Design review of the part shown in the three views and the two pictorial views. Dimensions are in mm from the part's minimum x, y and z. Give positions to 0.01 mm unless a question says otherwise; leave off trailing zeros. Loops run counter-clockwise (first coordinate to the right, second up) from the corner with the lowest first, then second, coordinate; pieces in that order, holes last.
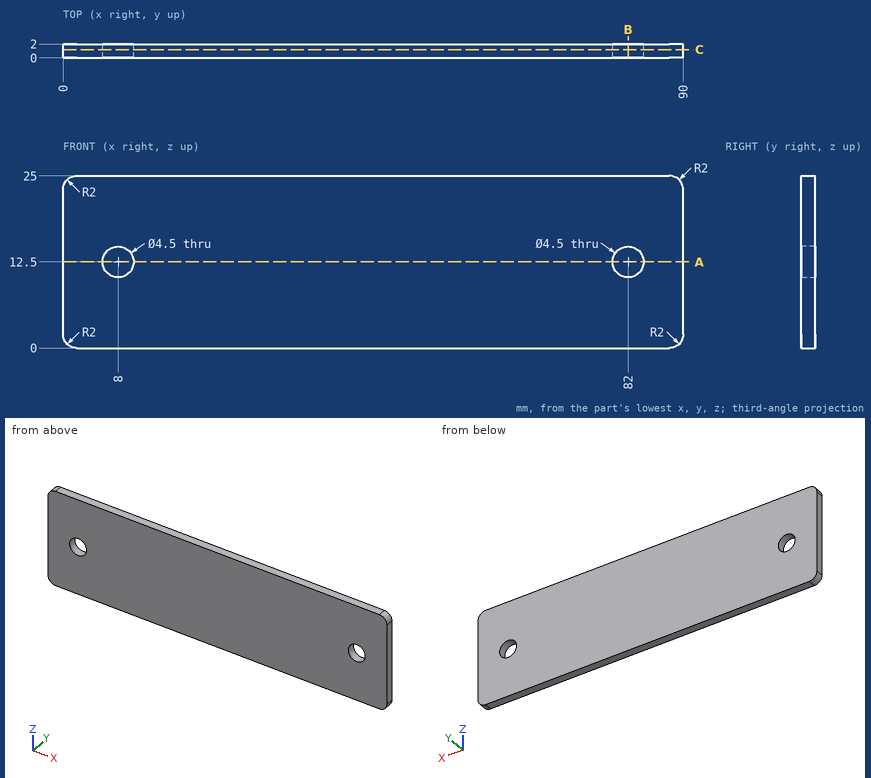
Q1. Consider section C-C on y = 1.2. Give the boundary of the cut face in (x, z).
Answers:
outline: (0, 2) arc R2 ccw to (2, 0) - (88, 0) arc R2 ccw to (90, 2) - (90, 23) arc R2 ccw to (88, 25) - (2, 25) arc R2 ccw to (0, 23) - close; hole circle Ø4.5 at (8, 12.5); hole circle Ø4.5 at (82, 12.5)
Q2. Consider section B-B on x = 82. Give the boundary of the cut face in (y, z), plus the area to 3 significant figures.
Answers:
outline: (0, 0) - (2, 0) - (2, 10.25) - (0, 10.25) - close; (0, 14.75) - (2, 14.75) - (2, 25) - (0, 25) - close
area: 41.0 mm2
Q3. For probe 1 along X at (y, z) = (0.6, 12.5); probe 2 along X at (y, z) = (1.05, 11.5); probe 3 along Z at (x, y) = (6, 0.25), list the stretches that pass through material, from the lowest coordinate up.
Answers:
probe 1: x = 0 to 5.75, 10.25 to 79.75, 84.25 to 90
probe 2: x = 0 to 5.98, 10.02 to 79.98, 84.02 to 90
probe 3: z = 0 to 11.47, 13.53 to 25
Q4. Consider section A-A on z = 12.5. Give the boundary of the cut face in (x, y), plus the area to 3 significant figures.
Answers:
outline: (0, 0) - (5.75, 0) - (5.75, 2) - (0, 2) - close; (10.25, 0) - (79.75, 0) - (79.75, 2) - (10.25, 2) - close; (84.25, 0) - (90, 0) - (90, 2) - (84.25, 2) - close
area: 162 mm2
Q5. For pin 1 Ø2.5 at (x, z) = (8, 12.5) entering from +Y, flat-tipped, find the tip position at first contact; note if it passes through.
Answers:
pin 1: passes through
